Study the drawing (mm; zero at the part's minimum x, y, z) and answer. Round coordinates to 2 decimals unless told otherwise and drop trailing zeros. Loops run counter-clockwise (first coordinate to the right, second up) from the corner with the lowest first, then second, coordinate; pieces in that order, holes last. Notation, with made-up numbers: M 62,79 L 70,79 A13 ccw 70,103 Z; hole C 38.5,80.25 d9. An arc over 180 degrees is marked long. Put each result on its own line as item: value. Start each with the question number.
(1) Section C-C, the plane y = 1.2 is taken. Determine the outline of the cut face in (x, z) (1 decimal).
(2) Straight lines are drawn through the part: line 1 (Z direction, x = 93.5, y = 0.7) (1 decimal); line 2 (X direction, y = 1.1, z = 26.5) (1 decimal). For each, find the intervals that lie inside material, in ascending order.
(3) A flat-ended cylindrical pin translates along its axis: P1, Ø13, axis at x = 93.5, z = 26.5, coming from the +Y side. Find the tip coordinate at first contact, or state that the pin passes through.
(4) Section B-B, the plane z = 26.5 is taken. Determine the outline of the cut face in (x, y) (1 decimal).
(5) Section A-A, the plane x = 93.5 is taken. Determine the outline of the cut face in (y, z) (1 decimal).
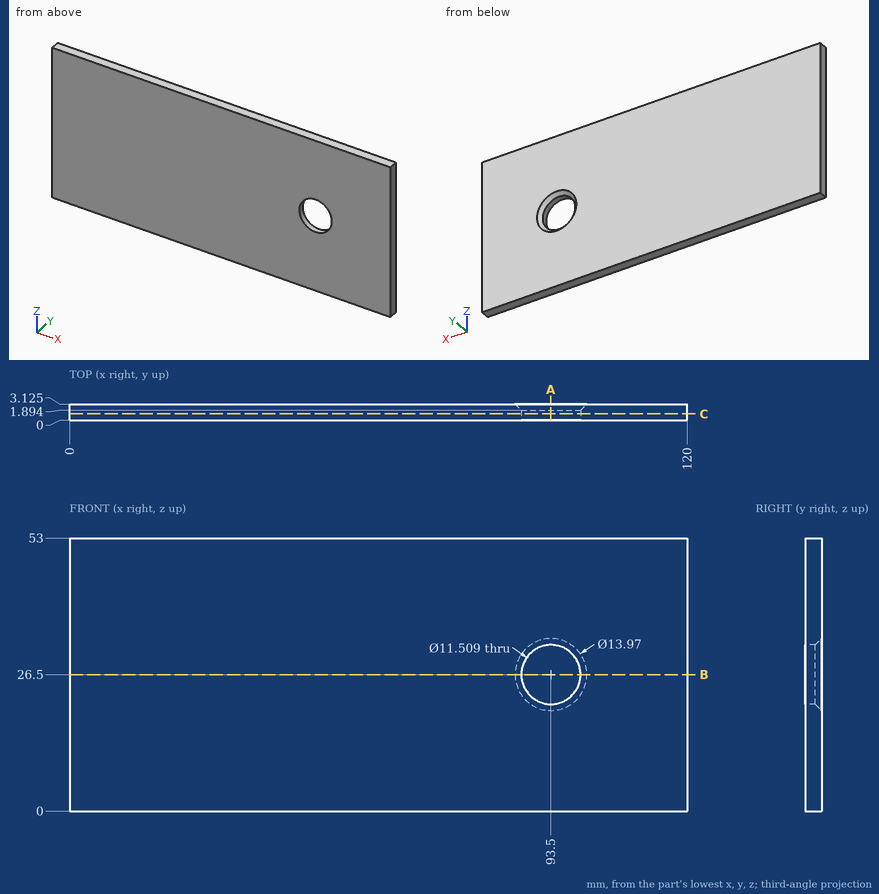
Recorded:
1. outline: M 0,0 L 120,0 L 120,53 L 0,53 Z; hole C 93.5,26.5 d11.5
2. line 1: z = 0 to 20.7, 32.3 to 53
2. line 2: x = 0 to 87.7, 99.3 to 120
3. P1: stops at y = 2.64
4. outline: M 0,0 L 87.7,0 L 87.7,1.9 L 86.5,3.1 L 0,3.1 Z; M 99.3,0 L 120,0 L 120,3.1 L 100.5,3.1 L 99.3,1.9 Z
5. outline: M 0,0 L 3.1,0 L 3.1,19.5 L 1.9,20.7 L 0,20.7 Z; M 0,32.3 L 1.9,32.3 L 3.1,33.5 L 3.1,53 L 0,53 Z
